```python
from build123d import *

# Parameters (mm, degrees)
MODEL_R             = 8
MODEL_R_2           = 1.5
MODEL_W             = 10
MODEL_H             = 3.5
MODEL_W_2           = 3.5
MODEL_H_2           = 10.5
MODEL_W_3           = 4.5
MODEL_W_4           = 35
MODEL_H_3           = 41
BOSS_EXTRUDE1_DEPTH = 3


with BuildPart() as part:
    # Model → Boss-Extrude1 (new body)
    with BuildSketch(Plane.XY):
        with BuildLine():
            Line((6.5, 3.5), (88.4, 3.5))
            ThreePointArc((88.4, 3.5), (95.471067812, 0.571067812), (98.4, -6.5))
            Line((98.4, -6.5), (98.4, -75.9))
            ThreePointArc((98.4, -75.9), (95.471067812, -82.971067812), (88.4, -85.9))
            Line((88.4, -85.9), (6.5, -85.9))
            ThreePointArc((6.5, -85.9), (-0.571067812, -82.971067812), (-3.5, -75.9))
            Line((-3.5, -75.9), (-3.5, -6.5))
            ThreePointArc((-3.5, -6.5), (-0.571067812, 0.571067812), (6.5, 3.5))
        make_face()
        with Locations((79.6, -20)):
            Circle(MODEL_R, mode=Mode.SUBTRACT)
        with Locations((79.6, -62.4)):
            Circle(MODEL_R, mode=Mode.SUBTRACT)
        with Locations((79.6, -41.2)):
            Circle(MODEL_R, mode=Mode.SUBTRACT)
        with Locations((46.5, -61.2)):
            Circle(MODEL_R_2, mode=Mode.SUBTRACT)
        with Locations((6.5, -21.2)):
            Circle(MODEL_R_2, mode=Mode.SUBTRACT)
        with Locations((72.4, -78.9)):
            Circle(MODEL_R_2, mode=Mode.SUBTRACT)
        with Locations((22.5, -3.5)):
            Circle(MODEL_R_2, mode=Mode.SUBTRACT)
        with Locations((72.4, -3.5)):
            Circle(MODEL_R_2, mode=Mode.SUBTRACT)
        with Locations((22.5, -78.9)):
            Circle(MODEL_R_2, mode=Mode.SUBTRACT)
        with Locations((6.5, -61.2)):
            Circle(MODEL_R_2, mode=Mode.SUBTRACT)
        with Locations((46.5, -21.2)):
            Circle(MODEL_R_2, mode=Mode.SUBTRACT)
        with Locations((59.4, -41.2)):
            Circle(MODEL_R, mode=Mode.SUBTRACT)
        with Locations((59.4, -62.4)):
            Circle(MODEL_R, mode=Mode.SUBTRACT)
        with Locations((59.4, -20)):
            Circle(MODEL_R, mode=Mode.SUBTRACT)
        with Locations((84.9, -79.15)):
            Rectangle(MODEL_W, MODEL_H, mode=Mode.SUBTRACT)
        with Locations((35, -79.15)):
            Rectangle(MODEL_W, MODEL_H, mode=Mode.SUBTRACT)
        with Locations((84.9, -3.25)):
            Rectangle(MODEL_W, MODEL_H, mode=Mode.SUBTRACT)
        with Locations((35, -3.25)):
            Rectangle(MODEL_W, MODEL_H, mode=Mode.SUBTRACT)
        with Locations((91.65, -41.2)):
            Rectangle(MODEL_W_2, MODEL_H_2, mode=Mode.SUBTRACT)
        with Locations((2.75, -41.2)):
            Rectangle(MODEL_W_3, MODEL_H_2, mode=Mode.SUBTRACT)
        with Locations((10, -3.25)):
            Rectangle(MODEL_W, MODEL_H, mode=Mode.SUBTRACT)
        with Locations((59.9, -3.25)):
            Rectangle(MODEL_W, MODEL_H, mode=Mode.SUBTRACT)
        with Locations((10, -79.15)):
            Rectangle(MODEL_W, MODEL_H, mode=Mode.SUBTRACT)
        with Locations((59.9, -79.15)):
            Rectangle(MODEL_W, MODEL_H, mode=Mode.SUBTRACT)
        with Locations((26.5, -41.2)):
            Rectangle(MODEL_W_4, MODEL_H_3, mode=Mode.SUBTRACT)
    extrude(amount=BOSS_EXTRUDE1_DEPTH)


solid = part.part
```
The listing builds one solid part. Answer for the finished solid, in the listing's coordinates (mm). Give positions to 0.01 mm unless a question says otherwise; leave off trailing zeros. Order: outer loops, then holes, each group sorted by start corner. A loop starts at its lowest first (then second) coordinate and runs counter-clockwise, first axis right, second up. Notation, with made-up numbers: (-20, 50) -> (1, 50) arc R24 cw to (1, 74) -> close; hole circle Ø6 at (8.25, -36.75). An arc over 180 degrees is marked (long way). Write each question's results on one line, items separated by ' | '.
Q1. The part is cut by section C-C, the plane y = -15. Give the vertices of the cut face in (x, z) (3 decimals).
Checked values:
outline: (-3.5, 0) -> (53.155, 0) -> (53.155, 3) -> (-3.5, 3) -> close; (65.645, 0) -> (73.355, 0) -> (73.355, 3) -> (65.645, 3) -> close; (85.845, 0) -> (98.4, 0) -> (98.4, 3) -> (85.845, 3) -> close
Q2. This flat-tipped pin is pushed along its axis until it touches: P1, Ø1.5, axis at y = -3, z = 1, coming from the +X side. Where does it stop, or does it pass through?
Checked values:
P1: stops at x = 98.01
Q3. The part is cut by section D-D, the plane x = 78. Give the vertices of the cut face in (y, z).
Checked values:
outline: (-85.9, 0) -> (-70.24, 0) -> (-70.24, 3) -> (-85.9, 3) -> close; (-54.56, 0) -> (-49.04, 0) -> (-49.04, 3) -> (-54.56, 3) -> close; (-33.36, 0) -> (-27.84, 0) -> (-27.84, 3) -> (-33.36, 3) -> close; (-12.16, 0) -> (3.5, 0) -> (3.5, 3) -> (-12.16, 3) -> close
Q4. The part is cut by section B-B, the plane x = 91. Give the vertices of the cut face in (y, z), and give its area (3 significant figures).
Checked values:
outline: (-85.56, 0) -> (-46.45, 0) -> (-46.45, 3) -> (-85.56, 3) -> close; (-35.95, 0) -> (3.16, 0) -> (3.16, 3) -> (-35.95, 3) -> close | area: 235 mm^2
Q5. Straight lines are drawn through the part: probe 1 along Y at (x, z) = (59.4, 2.3); probe 2 along Y at (x, z) = (22.5, 2.2); probe 3 along Y at (x, z) = (79.6, 1.7). For each, find the intervals that lie inside material, in ascending order. Write a range as from..to.
Checked values:
probe 1: y = -85.9..-80.9, -77.4..-70.4, -54.4..-49.2, -33.2..-28, -12..-5, -1.5..3.5 | probe 2: y = -85.9..-80.4, -77.4..-61.7, -20.7..-5, -2..3.5 | probe 3: y = -85.9..-70.4, -54.4..-49.2, -33.2..-28, -12..3.5
Q6. Determine the mould class of faces 1 (the face through (35, -77.4, 1)), 2 (the face through (-0.49, -83.05, 1.48)), 3 (the face through (48, -41, 3)) for opening direction Y: pulls with the +Y half, pulls with the -Y half, needs draft (parallel to the pull), parting line crosses it, or undercut.
Checked values:
face 1: undercut | face 2: pulls with the -Y half | face 3: needs draft
Q7. The part is cut by section A-A, the plane y = -51. Give the vertices of the cut face in (x, z).
Checked values:
outline: (-3.5, 0) -> (9, 0) -> (9, 3) -> (-3.5, 3) -> close; (44, 0) -> (98.4, 0) -> (98.4, 3) -> (44, 3) -> close
